Input: part model. Units: mm. Frame: model coordinates. A direction names the side the tool comes from. Coordinates: 2 decimals unless noted, no trailing zeros. Write each loop counter-clockwise with the first axis right and the second up, starting at its lowest first coordinate (ties: lowest second). Pieces come first, ordered by that corner, then holes. Notation, with made-up numbers: (88.5, -21) - (95.5, -21) arc R22 cw to (95.5, -9) - close; hole circle Ø1 at (-40, -36). An arc over 180 degrees is marked (long way). One line per question, with ' | ' between items. Start each with the question number.
1) Section query D-D on x = 3.5. Return loops of the section in (y, z) (3 decimals), and give its area (4 significant figures).
2) Line query: line 1 (Y direction, x = -19.05, z = 1.35); line 2 (X direction, y = -72, z = 1.9); line 3 (Y direction, x = 27, z = 2.55). Output: solid intervals per line, ascending.
3) Reachability of faces 1 (the flat face through (76.818, -89, 2)), 2 (the cylindrical face through (16.62, 4.87, 1.57)) from +Z, -Z, +X, -X, +Y, -Y: full face, straight path, thin tool, end or side. Return the list, or none.
4) Section query B-B on x = -19.05. Return loops of the section in (y, z) (3 decimals).
5) First-contact query: P1, Ø3, axis at x = 19.05, y = 4.1, coming from the +Z side; P2, Ø1.5, axis at x = 61.5, z = 2.5, coming from the +Y side; P3, Ø1.5, axis at y = -21.5, z = 1.5, coming from the +X side. Flat tips, straight axial feed; report the tip coordinate or a pass-through.
6) Section query A-A on y = -122.17. Return loops of the section in (x, z) (1 decimal), and give its area (3 significant figures).
7) Draft query along Y for faces 3 (the flat face through (62, -19, 3.175)), 4 (the flat face through (2, -15, 2)), 5 (the cylindrical face through (100.66, -120.06, 1.61)), 6 (the cylindrical face through (-17.026, 2.548, 1.565)). Return one class per face: released by +Y, released by -Y, zero draft, split by the parting line, or undercut.
8) Section query C-C on z = 0.6. Give the number of separate pieces and of enclosed holes in the cut face, and give its area (3 significant figures).
```python
from build123d import *

# Parameters (mm, degrees)
SKETCH1_W           = 76.2
SKETCH1_H           = 30
BOSS_EXTRUDE1_DEPTH = 3.175
BOSS_EXTRUDE2_DEPTH = 3.175
FILLET1_R           = 5
SKETCH5_R           = 2.5
CUT_EXTRUDE2_DEPTH  = 168.692302315
SKETCH6_R           = 2.55
CUT_EXTRUDE3_DEPTH  = 168.692302315
SKETCH7_R           = 2.55
CUT_EXTRUDE4_DEPTH  = 10


with BuildPart() as part:
    # Sketch1 → Boss-Extrude1 (new body)
    with BuildSketch(Plane.XY):
        Rectangle(SKETCH1_W, SKETCH1_H)
    extrude(amount=BOSS_EXTRUDE1_DEPTH)

    # Sketch3 → Boss-Extrude2 (add)
    with BuildSketch(Plane(origin=(0, 0, 0), x_dir=(-1, 0, 0), z_dir=(0, 0, -1))):
        with BuildLine():
            ThreePointArc((-38.1, 15), (-86.132736854, -5.252023618), (-106.8175, -53.1))
            Line((-106.8175, -53.1), (-106.8175, -129.230992121))
            Line((-106.8175, -129.230992121), (-76.8175, -129.230992121))
            Line((-76.8175, -129.230992121), (-76.8175, -53.1))
            ThreePointArc((-76.8175, -53.1), (-65.439370351, -25.940034949), (-38.1, -15))
            Line((-38.1, -15), (-38.1, 15))
        make_face()
    extrude(amount=-BOSS_EXTRUDE2_DEPTH)

    # Fillet1
    fillet1_edges = [part.edges().sort_by_distance(p)[0] for p in [
        (106.8175, -129.230992121, 1.5875),
        (76.8175, -129.230992121, 1.5875),
        (-38.1, 15, 1.5875),
        (-38.1, -15, 1.5875),
    ]]
    fillet(fillet1_edges, radius=FILLET1_R)

    # Sketch5 → Cut-Extrude2 (cut, through all)
    with BuildSketch(Plane.XY.offset(3.175)):
        with Locations((99.3175, -122.17)):
            Circle(SKETCH5_R)
        with Locations((84.3175, -122.17)):
            Circle(SKETCH5_R)
        with Locations((84.3175, -99.67)):
            Circle(SKETCH5_R)
        with Locations((99.3175, -99.67)):
            Circle(SKETCH5_R)
    extrude(amount=-CUT_EXTRUDE2_DEPTH, mode=Mode.SUBTRACT)

    # Sketch6 → Cut-Extrude3 (cut, through all)
    with BuildSketch(Plane(origin=(0, 0, 0), x_dir=(-1, 0, 0), z_dir=(0, 0, -1))):
        with Locations((-19.05, -8.6)):
            Circle(SKETCH6_R)
        with Locations((19.05, -8.6)):
            Circle(SKETCH6_R)
        with Locations((19.05, 4.1)):
            Circle(SKETCH6_R)
        with Locations((-19.05, 4.1)):
            Circle(SKETCH6_R)
    extrude(amount=-CUT_EXTRUDE3_DEPTH, mode=Mode.SUBTRACT)

    # Sketch7 → Cut-Extrude4 (cut)
    with BuildSketch(Plane(origin=(0, 0, 0), x_dir=(-1, 0, 0), z_dir=(0, 0, -1))):
        with Locations((-75.960370634, -15.248517141)):
            Circle(SKETCH7_R)
        with Locations((-91.8175, -53.1)):
            Circle(SKETCH7_R)
    extrude(amount=-CUT_EXTRUDE4_DEPTH, mode=Mode.SUBTRACT)


solid = part.part
```
Answer key:
1) outline: (-15, 0) - (15, 0) - (15, 3.175) - (-15, 3.175) - close | area: 95.25 mm²
2) line 1: -15 to -11.15, -6.05 to 1.55, 6.65 to 15 | line 2: 76.82 to 106.82 | line 3: -15 to 15
3) face 1: +Z, -Z, -X, -Y | face 2: +Z, -Z
4) outline: (-15, 0) - (-11.15, 0) - (-11.15, 3.175) - (-15, 3.175) - close; (-6.05, 0) - (1.55, 0) - (1.55, 3.175) - (-6.05, 3.175) - close; (6.65, 0) - (15, 0) - (15, 3.175) - (6.65, 3.175) - close
5) P1: through | P2: y = 10.82 | P3: x = 98.74
6) outline: (76.8, 0) - (81.8, 0) - (81.8, 3.2) - (76.8, 3.2) - close; (86.8, 0) - (96.8, 0) - (96.8, 3.2) - (86.8, 3.2) - close; (101.8, 0) - (106.8, 0) - (106.8, 3.2) - (101.8, 3.2) - close | area: 63.5 mm²
7) face 3: zero draft | face 4: released by -Y | face 5: undercut | face 6: undercut
8) separate pieces: 1 | enclosed holes: 10 | area: 6,820 mm²
